The listing builds one solid part. Answer for the finished solid, in the listing's coordinates (mm). A direction names the side the tool comes from. Coordinates: 2 decimals unless noted, no trailing zeros. Order: outer loops, then holes, each group sorted by start corner. A loop starts at its lowest first (then second) coordinate and runs counter-clockwise, first axis right, second up. Notation, with made-up numbers: (-16, 68) -> (37, 68) arc R32 cw to (37, 95) -> close; hole circle Ø11 at (-35.75, 73). An arc over 180 degrees is marked (long way). Return JSON: item names as keys, results as strings.
```python
from build123d import *

# Parameters (mm, degrees)
SKETCH_1_R               = 1.75
EXTRUDE_1_DEPTH          = 3
SKETCH_2_R               = 12.5
EXTRUDE_2_DEPTH          = 10
FILLET_1_R               = 2
SKETCH_5_R               = 10.5
EXTRUDE_4_DEPTH          = 30
SKETCH_7_W               = 18
SKETCH_7_H               = 40
EXTRUDE_5_DEPTH          = 28
CUT_EXTRUDE_1_DEPTH      = 70.036222376
CUT_EXTRUDE_1_DEPTH_BACK = 70.036222376
SHELL_START              = 17
SHELL_1_DEPTH            = 38
SHELL_START_2            = 2
SHELL_1_2_OUTLINE_R      = 8.5
SHELL_1_2_DEPTH          = 15
FILLET_2_R               = 10
SKETCH_9_R               = 2.5
CUT_EXTRUDE_2_DEPTH      = 70.036222376


# Read off the part's stored shape, not the designer's step: 抽壳1
with BuildPart() as part:
    # 草图1 → 凸台-拉伸1 (new body)
    with BuildSketch(Plane.XY):
        with BuildLine():
            Line((-14, -17.5), (14, -17.5))
            ThreePointArc((14, -17.5), (18.242640687, -15.742640687), (20, -11.5))
            Line((20, -11.5), (20, 11.5))
            ThreePointArc((20, 11.5), (18.242640687, 15.742640687), (14, 17.5))
            Line((14, 17.5), (-14, 17.5))
            ThreePointArc((-14, 17.5), (-18.242640687, 15.742640687), (-20, 11.5))
            Line((-20, 11.5), (-20, -11.5))
            ThreePointArc((-20, -11.5), (-18.242640687, -15.742640687), (-14, -17.5))
        make_face()
        with Locations((-14.285714286, 12.5)):
            Circle(SKETCH_1_R, mode=Mode.SUBTRACT)
        with Locations((-14.285714286, -12.5)):
            Circle(SKETCH_1_R, mode=Mode.SUBTRACT)
        with Locations((14.285714286, -12.5)):
            Circle(SKETCH_1_R, mode=Mode.SUBTRACT)
        with Locations((14.285714286, 12.5)):
            Circle(SKETCH_1_R, mode=Mode.SUBTRACT)
    extrude(amount=EXTRUDE_1_DEPTH)

    # 草图2 → 凸台-拉伸2 (add)
    with BuildSketch(Plane.XY.offset(3)):
        with Locations(Location((0, 0, 0), (0, 0, 180))):
            Circle(SKETCH_2_R)
    extrude(amount=EXTRUDE_2_DEPTH)

    # 圆角1
    fillet_1_edges = [part.edges().sort_by_distance(p)[0] for p in [
        (12.5, 0, 13),
    ]]
    fillet(fillet_1_edges, radius=FILLET_1_R)

    # 草图5 → 凸台-拉伸4 (add)
    with BuildSketch(Plane.XY.offset(13)):
        Circle(SKETCH_5_R)
    extrude(amount=EXTRUDE_4_DEPTH)

    # Surface Cut 2
    split(bisect_by=Plane(origin=(0, -15.906854249, 15.906854249), x_dir=(1, 0, 0), z_dir=(0, -0.7071067811865488, 0.7071067811865464)), keep=Keep.BOTTOM)

    # 草图7 → 凸台-拉伸5 (add)
    with BuildSketch(Plane(origin=(0, 30, 0), x_dir=(1, 0, 0), z_dir=(0, 1, 0))):
        with Locations((0, -35)):
            Rectangle(SKETCH_7_W, SKETCH_7_H)
    extrude(amount=-EXTRUDE_5_DEPTH)

    # 草图8 → 切除-拉伸1 (cut, two sides: drawn at the far end of the back side and taken through both)
    with BuildSketch(Plane(origin=(9, 0, 0), x_dir=(0, 0, -1), z_dir=(1, 0, 0)).offset(-CUT_EXTRUDE_1_DEPTH_BACK)):
        Polygon((-37.222035412, 5.408326913), (-55, 5.408326913), (-55, 2), (-33.813708499, 2), align=None)
    extrude(amount=CUT_EXTRUDE_1_DEPTH + CUT_EXTRUDE_1_DEPTH_BACK, mode=Mode.SUBTRACT)

    # 抽壳1 outline → 抽壳1 (cut)
    with BuildSketch(Plane.XY.offset(SHELL_START)):
        with BuildLine():
            Line((7, 30), (-7, 30))
            Line((-7, 30), (-7, 4.82182538))
            ThreePointArc((-7, 4.82182538), (0, -8.5), (7, 4.82182538))
            Line((7, 4.82182538), (7, 30))
        make_face()
    extrude(amount=SHELL_1_DEPTH, mode=Mode.SUBTRACT)

    # Shell 1 2 outline → Shell 1 2 (cut)
    with BuildSketch(Plane.XY.offset(SHELL_START_2)):
        Circle(SHELL_1_2_OUTLINE_R)
    extrude(amount=SHELL_1_2_DEPTH, mode=Mode.SUBTRACT)

    # 圆角2
    fillet_2_edges = [part.edges().sort_by_distance(p)[0] for p in [
        (8, 5.408326913, 55),
        (8, 30, 55),
        (-8, 30, 55),
        (-8, 5.408326913, 55),
    ]]
    fillet(fillet_2_edges, radius=FILLET_2_R)

    # 草图9 → 切除-拉伸2 (cut, through all)
    with BuildSketch(Plane(origin=(9, 0, 0), x_dir=(0, 0, -1), z_dir=(1, 0, 0))):
        with Locations((-50, 17.704163457)):
            Circle(SKETCH_9_R)
    extrude(amount=-CUT_EXTRUDE_2_DEPTH, mode=Mode.SUBTRACT)


solid = part.part
```
Item 1: Which of the six approach directions +Z, -Z, +X, -X, +Y, -Y give full straight-line access (tool end or side, diameter ignored) to faces 1 (the flat face through (0, 18, 17)), 2 (the flat face through (9, 18, 35)), 3 (the flat face through (-7.4, 30, 26.6)), 4 (the flat face through (0, 17.5, 1)), 5 (the flat face through (8, 5.408, 41))?
Answer list:
{"face 1": "+Z, +Y", "face 2": "+Z, +X, +Y", "face 3": "+Z, -Z, +X, -X, +Y", "face 4": "-Z, +X, -X, +Y", "face 5": "+Z, +X, -X, -Y"}
Item 2: Flat-ended cylindrical pins translate along their axes: pin 1 (5.5 mm diameter, centred on x = 2, y = 21, fed in from -Z); pin 2 (10 mm diameter, centred on y = 10.5, z = 46.5, fed in from -X); pin 3 (0.9 mm diameter, centred on x = -4.5, z = 2, fed in from +Y); pin 4 (15.5 mm diameter, centred on x = 3.5, y = 16, fed in from +Z). Find the tip coordinate at first contact, or state that the pin passes through.
Answer list:
{"pin 1": "z = 15", "pin 2": "x = -9", "pin 3": "y = 17.5", "pin 4": "z = 55"}
Item 3: The part is cut by section A-A on z = 25. Determine the outline of the cut face in (x, y), plus the area to 3 significant figures.
Answer list:
{"outline": "(-9, 5.41) arc R10.5 ccw to (-7.99, -6.81) -> (-5.08, -6.81) arc R8.5 cw to (-7, 4.82) -> (-7, 30) -> (-9, 30) -> close; (5.08, -6.81) -> (7.99, -6.81) arc R10.5 ccw to (9, 5.41) -> (9, 30) -> (7, 30) -> (7, 4.82) arc R8.5 cw to start", "area": "152 mm2"}
Item 4: The part is cut by section B-B on x = 0. Determine the outline of the cut face in (y, z).
Answer list:
{"outline": "(-17.5, 0) -> (17.5, 0) -> (17.5, 3) -> (12.5, 3) -> (12.5, 11) arc R2 ccw to (10.5, 13) -> (10.5, 15) -> (30, 15) -> (30, 17) -> (8.5, 17) -> (8.5, 2) -> (-8.5, 2) -> (-8.5, 23.31) -> (-10.5, 21.31) -> (-10.5, 13) arc R2 ccw to (-12.5, 11) -> (-12.5, 3) -> (-17.5, 3) -> close"}
Item 5: Find the intervals of material crossed by probe 1 along X at (y, z) = (14, 30.5); probe 2 along X at (y, z) = (0, 27.5); probe 3 along X at (y, z) = (-12, 2), in increasing order.
Answer list:
{"probe 1": "-9 to -7, 7 to 9", "probe 2": "-10.5 to -8.5, 8.5 to 10.5", "probe 3": "-19.98 to -15.96, -12.61 to 12.61, 15.96 to 19.98"}
Item 6: The part is cut by section C-C on z = 50. Determine the outline of the cut face in (x, y), plus the area to 3 significant figures.
Answer list:
{"outline": "(-9, 6.75) -> (-7, 6.75) -> (-7, 15.2) -> (-9, 15.2) -> close; (-9, 20.2) -> (-7, 20.2) -> (-7, 28.66) -> (-9, 28.66) -> close; (7, 6.75) -> (9, 6.75) -> (9, 15.2) -> (7, 15.2) -> close; (7, 20.2) -> (9, 20.2) -> (9, 28.66) -> (7, 28.66) -> close", "area": "67.6 mm2"}
Item 7: Determine the mould class of faces 6 (the flat face through (-8, 18, 55)), 7 (the cylindrical face through (18.289, 15.696, 1.479)), 8 (the flat face through (0, 0, 2)), 9 (the cylindrical face through (-15.58, -11.32, 1.48)) for opening direction X: pulls with the +X half, pulls with the -X half, needs draft (parallel to the pull), parting line crosses it, or undercut.
Answer list:
{"face 6": "needs draft", "face 7": "pulls with the +X half", "face 8": "undercut", "face 9": "undercut"}
Item 8: The part is cut by section D-D on y = 0. Determine the outline of the cut face in (x, z), plus the area to 3 significant figures.
Answer list:
{"outline": "(-20, 0) -> (20, 0) -> (20, 3) -> (12.5, 3) -> (12.5, 11) arc R2 ccw to (10.5, 13) -> (10.5, 31.81) -> (8.5, 31.81) -> (8.5, 2) -> (-8.5, 2) -> (-8.5, 31.81) -> (-10.5, 31.81) -> (-10.5, 13) arc R2 ccw to (-12.5, 11) -> (-12.5, 3) -> (-20, 3) -> close", "area": "257 mm2"}
